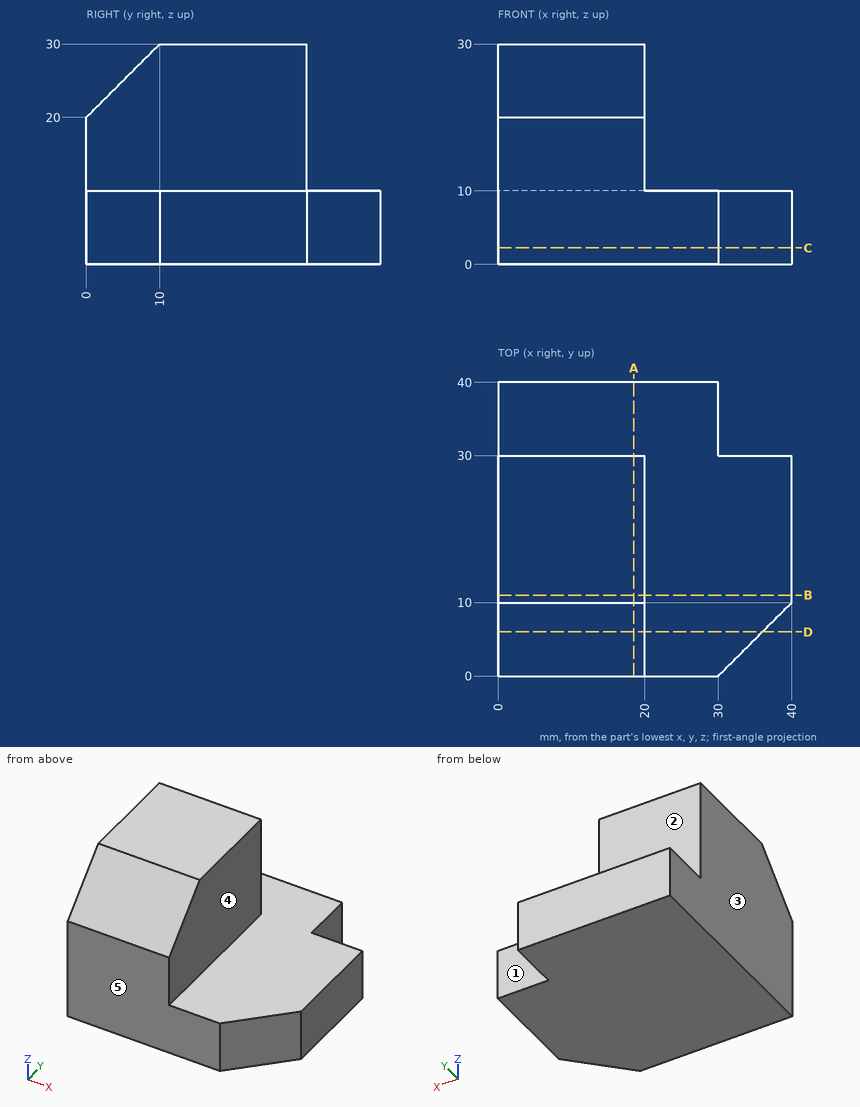
Job drawing, mm, ordinate dimensions from the low corner. One solid piece. A direction names the side the tool comes from. Round coordinates to 2 decimals unless told otherwise and drop trailing zeros. Order: outer loops, then holes, each group sorted by start corner. A loop starts at its lowest first (then second) coordinate and runs counter-clockwise, first axis right, second up. Notation, with made-up numbers: (58, -15.75) -> (93, -15.75) arc R28 cw to (93, 3.25) -> close; hole circle Ø9 at (-39.5, 86.25). An arc over 180 degrees is marked (long way). Answer in a Markdown table with one row per item.
1) Band-saw the part on D-D on y = 6. Give the cut face in (x, z).
Values:
| item | result |
|---|---|
| outline | (0, 0) -> (36, 0) -> (36, 10) -> (20, 10) -> (20, 26) -> (0, 26) -> close |
2) Pin check, flat tips, straight feed: P1, Ø8, axis at x = 18, z = 22.5, coming from the +Y side; P2, Ø1, axis at y = 27.5, z = 19, coming from the +X side; P3, Ø3, axis at x = 29.5, y = 33, coming from the +Z side. Stop position of each tip, or through.
Values:
| item | result |
|---|---|
| P1 | y = 30 |
| P2 | x = 20 |
| P3 | z = 10 |
3) Wall check: L1, parallel to X at y = 27.5, z = 18.5; L2, parallel to Z at x = 30.5, y = 5.5; L3, parallel to Y at x = 2, z = 14.75. Give the ranges that are in metal, low to high.
Values:
| item | result |
|---|---|
| L1 | 0 to 20 |
| L2 | 0 to 10 |
| L3 | 0 to 30 |
4) Band-saw the part on A-A on x = 18.5. Give the cut face in (y, z).
Values:
| item | result |
|---|---|
| outline | (0, 0) -> (40, 0) -> (40, 10) -> (30, 10) -> (30, 30) -> (10, 30) -> (0, 20) -> close |
5) Band-saw the part on B-B on y = 11. Give the cut face in (x, z).
Values:
| item | result |
|---|---|
| outline | (0, 0) -> (40, 0) -> (40, 10) -> (20, 10) -> (20, 30) -> (0, 30) -> close |
6) Band-saw the part on C-C on z = 2.25. Give the cut face in (x, y).
Values:
| item | result |
|---|---|
| outline | (0, 0) -> (30, 0) -> (40, 10) -> (40, 30) -> (30, 30) -> (30, 40) -> (0, 40) -> close |
7) Which spindle directions (+Z, -Z, +X, -X, +Y, -Y) get a long thin tool onto all of the face, cutting with end or side? Do the marked faces 1, 2, 3, 4 and 5. Say none if no direction does.
Values:
| item | result |
|---|---|
| face 1 | +Z, -Z, +X, +Y |
| face 2 | +Z, +X, -X, +Y |
| face 3 | +Z, -Z, -X, +Y, -Y |
| face 4 | +Z, +X, +Y, -Y |
| face 5 | +Z, -Z, +X, -X, -Y |
